Can you work these out from the model? Positions are in its coordinate system, mm. A direction names the side the tool comes from. Give positions to 0.01 mm unless a question says otherwise; leave off trailing zeros. Order: outer loops, then holes, each group sorted by start corner. A loop starts at its lowest first (then second) coordinate and runs counter-clockwise, first axis right, second up. Notation, with made-up numbers: M -3,19.5 L 55,19.5 A23 ccw 55,41.5 Z; hole C 0,-31 d1. An arc over 180 degrees is marked long. Answer as a JSON object with one key per item and string values.
```python
from build123d import *

# Parameters (mm, degrees)
F0_W     = 38.1
F0_H     = 38.1
F0_W_2   = 28.5496
F0_H_2   = 28.5496
F1_DEPTH = 914.4
F4_DEPTH = 38.101
F5_DEPTH = 38.101


with BuildPart() as f1:
    # F0 (on Front) → F1 (new body)
    with BuildSketch(Plane.XZ):
        Rectangle(F0_W, F0_H)
        Rectangle(F0_W_2, F0_H_2, mode=Mode.SUBTRACT)
    extrude(amount=F1_DEPTH)

    # F2 (on face) → F4 (cut, through all)
    with BuildSketch(Plane.XY.offset(19.05)):
        Polygon((19.05, 0), (-19.05, 0), (19.05, -38.1), align=None)
    extrude(amount=-F4_DEPTH, mode=Mode.SUBTRACT)

    # F3 (on face) → F5 (cut, through all)
    with BuildSketch(Plane(origin=(-19.05, 0, 0), x_dir=(0, -1, 0), z_dir=(-1, 0, 0))):
        Polygon((876.3, 19.05), (914.4, -19.05), (914.4, 19.05), align=None)
    extrude(amount=-F5_DEPTH, mode=Mode.SUBTRACT)


solid = f1.part
```
1) I want a section at A-A on z = 1. Write out the boundary of the cut face in (x, y), and give its area (3 significant figures).
Results found:
{"outline": "M -19.05,-894.35 L -14.27,-894.35 L -14.27,-4.78 L -19.05,0 Z; M 14.27,-894.35 L 19.05,-894.35 L 19.05,-38.1 L 14.27,-33.32 Z", "area": "8,360 mm²"}
2) I want a section at C-C on y = -289.5. Write out the boundary of the cut face in (x, z).
Results found:
{"outline": "M -19.05,-19.05 L 19.05,-19.05 L 19.05,19.05 L -19.05,19.05 Z; hole M -14.27,-14.27 L 14.27,-14.27 L 14.27,14.27 L -14.27,14.27 Z"}
3) For faces 4 (the face through (0, -437, 14.275)), 5 (the face through (-19.05, -451, 0)), which set-ups out of +Z, -Z, +X, -X, +Y, -Y let a thin tool reach every point of the face, with its end or its side?
Results found:
{"face 4": "+Y, -Y", "face 5": "+Z, -Z, -X, +Y, -Y"}
4) I'm going to push a flat-ended pin straight in: pin 1 Ø5 at (x, z) = (-13.5, 3) entering from +Y. Where does the tip first touch, or does it pass through?
Results found:
{"pin 1": "stops at y = -3.05"}
5) Thinking about a two-plate mould opening in X: for faces 1 (the face through (16.67, -895.08, 0.27)), 2 (the face through (-0.27, -18.78, -16.67)), 3 (the face through (0, -451, -14.275)), which applies, pulls with the +X half, pulls with the -X half, needs draft (parallel to the pull), parting line crosses it, or undercut?
Results found:
{"face 1": "needs draft", "face 2": "pulls with the +X half", "face 3": "undercut"}
6) I want a section at B-B on x = -5. Write out the boundary of the cut face in (y, z).
Results found:
{"outline": "M -914.4,-19.05 L -14.05,-19.05 L -14.05,-14.27 L -909.62,-14.27 Z; M -881.08,14.27 L -14.05,14.27 L -14.05,19.05 L -876.3,19.05 Z"}
7) I need wall thicknesses on L1, parallel to Z at x = 12.5, y = -838.5; L2, parallel to Y at x = 15.5, z = -1. Which ranges of each line are inside material? Lowest first, please.
Results found:
{"L1": "z = -19.05 to -14.27, 14.27 to 19.05", "L2": "y = -896.35 to -34.55"}
